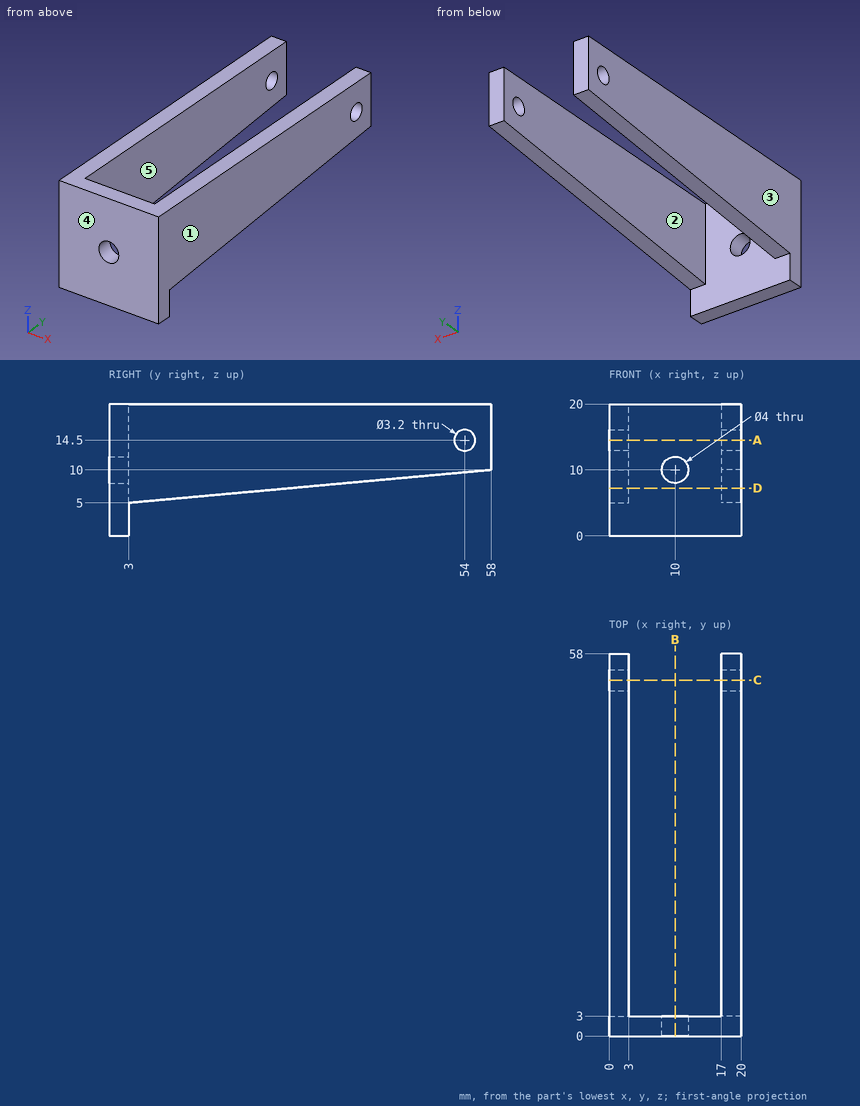
Input: dimensioned drawing with shaded views. Units: mm. Origin: part minimum x, y, z. A direction names the side the tool comes from. Give positions to 0.01 mm unless a question says otherwise; leave off trailing zeros. Order: outer loops, then holes, each group sorted by start corner. A loop starts at its lowest first (then second) coordinate and runs counter-clockwise, first axis right, second up.
(1) Section query C-C (y = 54). Return the cut outline in (x, z), plus the area to 3 significant figures.
(2) Section query B-B (x = 10). Return the cut outline in (y, z), plus the area to 3 significant figures.
(3) Material intervals for line 1 along X through (y, z) = (39.5, 18.75); line 2 along Y through (x, z) = (1.7, 14.5); line 3 along Z through (x, y) = (10, 1.2), sorted ascending.
(4) Access query for the marked faces 1 and 2. Directions: +Z, -Z, +X, -X, +Y, -Y. A direction counts if a zero-diameter tool reaches every point of the face in a straight line with its end or side. Return the directions, or none.
(5) Pull-direction query (X, two-part tool) for the marked faces 3, 4 and 5; classes: +X half, -X half, draft (parallel to the pull), parting line (faces both ways), or undercut.
(6) Contact query for flat-ended pins moving along their axis: P1, Ø3, axis at x = 10, z = 10, coming from the +Y side; P2, Ø4, axis at x = 11, z = 7, coming from the +Y side; P3, Ø12, axis at x = 2.5, y = 16.5, coming from the -Z side. Output: stop coordinate, or through.
(7) Section query D-D (z = 7.25). Return the cut outline in (x, y).
(8) Section query A-A (z = 14.5). Return the cut outline in (x, y), plus the area to 3 significant figures.
Outcome:
1. outline: (0, 9.64) - (3, 9.64) - (3, 12.9) - (0, 12.9) - close; (0, 16.1) - (3, 16.1) - (3, 20) - (0, 20) - close; (17, 9.64) - (20, 9.64) - (20, 12.9) - (17, 12.9) - close; (17, 16.1) - (20, 16.1) - (20, 20) - (17, 20) - close
1. area: 43.0 mm2
2. outline: (0, 0) - (3, 0) - (3, 8) - (0, 8) - close; (0, 12) - (3, 12) - (3, 20) - (0, 20) - close
2. area: 48.0 mm2
3. line 1: x = 0 to 3, 17 to 20
3. line 2: y = 0 to 52.4, 55.6 to 58
3. line 3: z = 0 to 8, 12 to 20
4. face 1: +Z, -Z, +X, +Y, -Y
4. face 2: +Z, -Z, +Y
5. face 3: -X half
5. face 4: draft
5. face 5: undercut
6. P1: passes through
6. P2: stops at y = 3
6. P3: stops at z = 5.68
7. outline: (0, 0) - (20, 0) - (20, 27.75) - (17, 27.75) - (17, 3) - (3, 3) - (3, 27.75) - (0, 27.75) - close
8. outline: (0, 0) - (20, 0) - (20, 52.4) - (17, 52.4) - (17, 3) - (3, 3) - (3, 52.4) - (0, 52.4) - close; (0, 55.6) - (3, 55.6) - (3, 58) - (0, 58) - close; (17, 55.6) - (20, 55.6) - (20, 58) - (17, 58) - close
8. area: 371 mm2
